Here's how the part is built. I have some questions about the finished solid (model axes, mm). Coordinates: 2 decimals unless noted, no trailing zeros. Loops run counter-clockwise (first coordinate to the right, second up) from the corner with the lowest first, then second, coordinate; pieces in that order, holes last. Notation, with made-up numbers: M 82,26.25 L 122,26.25 A29 cw 122,60.25 Z; hole C 12.25,34 d2. An arc over 180 degrees is marked long. Use one line per item in the form item = value. Start each with the question number.
(1) Imagine slicing it at C-C, the plane z = 480. Please give me the cut outline in (x, y).
(2) Imagine slicing it at A-A, the plane y = 16. Please give me the cut outline in (x, z).
(3) Imagine slicing it at D-D, the plane z = 228. Please give me the cut outline in (x, y).
(4) Please list where these lines run through material, in increasing order: L1, parallel to Z at x = 173, y = 16; L2, parallel to Y at x = 474.5, z = 166; L3, parallel to Z at x = 267, y = 23.5.
(5) Imagine slicing it at B-B, the plane x = 640. Please give me the cut outline in (y, z).
(6) Will these pins go through, and if not, where does the flat tip stop? P1, Ø3, axis at y = -0.5, z = 20.5, coming from the +X side; P2, Ø1.5, axis at y = 16, z = 370, coming from the -X side; P3, Ø4, axis at y = 9.5, z = 218, coming from the -X side.
```python
from build123d import *

# Parameters (mm, degrees)
SKETCH1_R               = 48
BOSS_EXTRUDE1_DEPTH     = 32
SKETCH2_R               = 32
SKETCH2_R_2             = 24
BOSS_EXTRUDE2_DEPTH     = 32
BOSS_EXTRUDE3_START     = 32
SKETCH3_R               = 32
SKETCH3_R_2             = 24
BOSS_EXTRUDE3_DEPTH     = 32
CUT_EXTRUDE1_DEPTH      = 32
CUT_EXTRUDE1_DEPTH_BACK = 689
SKETCH4_R               = 24


with BuildPart() as part:
    # Sketch1 → Boss-Extrude1 (new body)
    with BuildSketch(Plane(origin=(0, 0, 0), x_dir=(1, 0, 0), z_dir=(0, 1, 0))):
        with BuildLine():
            ThreePointArc((64, 0), (-51.919499851, 37.421458218), (20.238577025, -60.715731075))
            Line((20.238577025, -60.715731075), (160, -480))
            Line((160, -480), (480, -480))
            Line((480, -480), (619.761422975, -60.715731075))
            ThreePointArc((619.761422975, -60.715731075), (691.919499851, 37.421458218), (576, 0))
            Line((576, 0), (64, 0))
        make_face()
        with Locations(Location((0, 0, 0), (0, 0, 270))):
            Circle(SKETCH1_R, mode=Mode.SUBTRACT)
        with Locations(Location((640, 0, 0), (0, 0, 270))):
            Circle(SKETCH1_R, mode=Mode.SUBTRACT)
    extrude(amount=BOSS_EXTRUDE1_DEPTH)

    # Sketch2 → Boss-Extrude2 (add)
    with BuildSketch(Plane(origin=(160, 0, 0), x_dir=(0, -1, 0), z_dir=(-1, 0, 0))):
        with Locations((-16, 480)):
            Circle(SKETCH2_R)
        with Locations((-16, 480)):
            Circle(SKETCH2_R_2, mode=Mode.SUBTRACT)
    extrude(amount=-BOSS_EXTRUDE2_DEPTH)

    # Sketch3 → Boss-Extrude3 (add)
    with BuildSketch(Plane(origin=(480, 0, 0), x_dir=(0, -1, 0), z_dir=(-1, 0, 0)).offset(BOSS_EXTRUDE3_START)):
        with Locations((-16, 480)):
            Circle(SKETCH3_R)
        with Locations((-16, 480)):
            Circle(SKETCH3_R_2, mode=Mode.SUBTRACT)
    extrude(amount=-BOSS_EXTRUDE3_DEPTH)

    # Sketch4 → Cut-Extrude1 (cut, two sides: drawn at the far end of the back side and taken through both)
    with BuildSketch(Plane(origin=(160, 0, 0), x_dir=(0, -1, 0), z_dir=(-1, 0, 0)).offset(-CUT_EXTRUDE1_DEPTH_BACK)):
        with Locations(Location((-16, 480, 0), (0, 0, 228.189685104))):
            Circle(SKETCH4_R)
    extrude(amount=CUT_EXTRUDE1_DEPTH + CUT_EXTRUDE1_DEPTH_BACK, mode=Mode.SUBTRACT)


solid = part.part
```
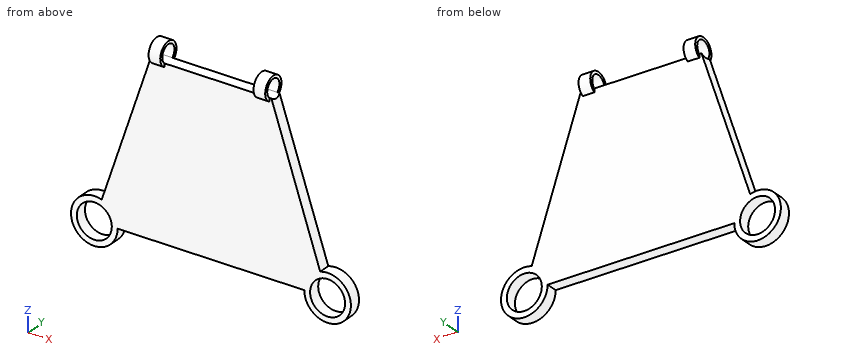
Answer:
q1.outline = M 160,-16 L 192,-16 L 192,-8 L 160,-8 Z; M 160,40 L 192,40 L 192,48 L 160,48 Z; M 448,-16 L 480,-16 L 480,-8 L 448,-8 Z; M 448,40 L 480,40 L 480,48 L 448,48 Z
q2.outline = M 20.24,60.72 A64 ccw long 64,0 L 576,0 A64 ccw long 619.76,60.72 L 488,456 L 152,456 Z; M 160,504 L 192,504 L 192,512 L 160,512 Z; M 448,504 L 480,504 L 480,512 L 448,512 Z; hole C 0,0 d96; hole C 640,0 d96
q3.outline = M 76,0 L 564,0 L 564,32 L 76,32 Z
q4.L1 = 0 to 456, 504 to 512
q4.L2 = 0 to 32
q4.L3 = 0 to 457.2
q5.outline = M 0,-64 L 32,-64 L 32,-48 L 0,-48 Z; M 0,48 L 32,48 L 32,64 L 0,64 Z
q6.P1 = 701.09
q6.P2 = 123.08
q6.P3 = 72
